The figure shows three views and two pictorial views of one solid part (mm, origin at its lowest corner). Answer the questions. Coordinates: 2 decimals unless noted, no trailing zeros. Write each loop counter-clockwise with the first axis right and the second up, starting at its lowest first coordinate (ties: lowest second). Pieces come first, ordered by that corner, then holes. Notation, with made-up numbers: M 85.25,40.25 L 134.25,40.25 A15 cw 134.25,49.25 Z; hole C 54.5,4.5 d9. An arc over 180 degrees is marked long. Use a Markdown table: item, result. Add a question column.
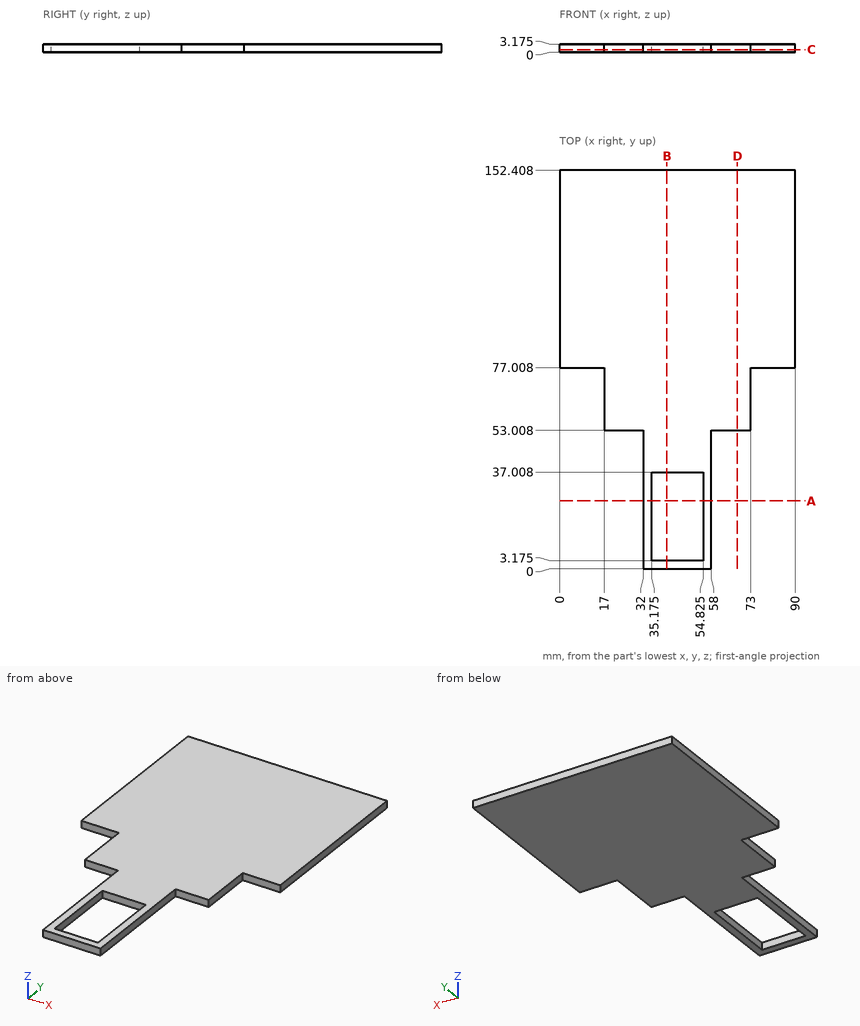
Item 1: Find section C-C on z = 1.05. Give the vertices of the cut face in (x, y) (1 decimal).
Item 2: Consider probe 1 along X at (y, z) = (21, 1.45) (3 decimals); probe 2 along Y at (x, z) = (47, 2.1) (1 decimal); probe 3 along Y at (x, z) = (65, 0.6). Determine where each line is inside the solid, lowest interval first.
Item 3: Each of these flat-tipped pins is pushed along its axis until it touches: pin 1 (1.6 mm diameter, centred on y = 16, z = 1, fed in from +X); pin 2 (1.6 mm diameter, centred on x = 78, z = 1.5, fed in from -Y); pin 3 (1 mm diameter, centred on y = 59.5, z = 1, fed in from -X). Where does it stop, or does it pass through?
Item 4: Find section D-D on x = 68. Give the vertices of the cut face in (y, z) (1 decimal), then the cut area to 3 significant figures.
Item 5: Find section A-A on y = 26. Give the vertices of the cut face in (x, z) (3 decimals).
Item 6: Find section B-B on x = 41. Give the vertices of the cut face in (y, z) (1 decimal).
Geometry says:
| question | item | result |
|---|---|---|
| 1 | outline | M 0,77 L 17,77 L 17,53 L 32,53 L 32,0 L 58,0 L 58,53 L 73,53 L 73,77 L 90,77 L 90,152.4 L 0,152.4 Z; hole M 35.2,3.2 L 54.8,3.2 L 54.8,37 L 35.2,37 Z |
| 2 | probe 1 | x = 32 to 35.175, 54.825 to 58 |
| 2 | probe 2 | y = 0 to 3.2, 37 to 152.4 |
| 2 | probe 3 | y = 53.01 to 152.41 |
| 3 | pin 1 | stops at x = 58 |
| 3 | pin 2 | stops at y = 77.01 |
| 3 | pin 3 | stops at x = 17 |
| 4 | outline | M 53,0 L 152.4,0 L 152.4,3.2 L 53,3.2 Z |
| 4 | area | 316 mm2 |
| 5 | outline | M 32,0 L 35.175,0 L 35.175,3.175 L 32,3.175 Z; M 54.825,0 L 58,0 L 58,3.175 L 54.825,3.175 Z |
| 6 | outline | M 0,0 L 3.2,0 L 3.2,3.2 L 0,3.2 Z; M 37,0 L 152.4,0 L 152.4,3.2 L 37,3.2 Z |
